Geometry check sheet. Reference: the model listing, model coordinates, mm. Face numbers are marked on the shaded views. A direction names the side the tool comes from. Give positions to 0.01 mm unless a question says otherwise; leave off trailing zeros. Write each loop counter-clockwise with the first axis right and the second up, starting at its lowest first coordinate (ties: lowest second). Pieces come first, ordered by that corner, then holes. Notation, with made-up numbers: M -37.5,18 L -32.5,18 A30 ccw -32.5,52 Z; hole C 19.25,74 d4. An arc over 180 degrees is marked long. Use one line per item in the form item = value. Start each with the question number.
```python
from build123d import *

# Parameters (mm, degrees)
F1_DEPTH  = 11.5
F3_R      = 2.75
F3_R_2    = 2.1
F4_DEPTH  = 7.2
F4_TAPER  = 1
F5_W      = 8.4
F5_H      = 28
F6_DEPTH  = 8
F8_DEPTH  = 15
F10_W     = 4.6
F10_H     = 5.4
F11_DEPTH = 20
F12_W     = 10.3
F12_H     = 7.2
F13_DEPTH = 10
F14_R     = 2
F15_DEPTH = 2
F16_R     = 2.1
F17_DEPTH = 2
F18_R     = 2.1
F19_DEPTH = 2
F20_R     = 2.1
F21_DEPTH = 2
F22_R     = 2.1
F23_DEPTH = 2
F24_R     = 2.1
F25_DEPTH = 2
F26_W     = 10.3
F26_H     = 7.2
F27_DEPTH = 10
F9_R      = 1.75
F28_DEPTH = 12
F29_R     = 1.5
F30_DEPTH = 0.8
F31_W     = 4.9
F31_H     = 8
F32_DEPTH = 1
F33_W     = 3
F33_H     = 1
F34_DEPTH = 5
F35_W     = 3
F35_H     = 1
F36_DEPTH = 5


with BuildPart() as f1:
    # F0 (on Front) → F1 (new body)
    with BuildSketch(Plane.XZ):
        Polygon((0.1941817731, -9.3541857075), (0.1941817731, 10.6458142925), (-6.1058182269, 10.6458142925), (-6.1058182269, 3.3958142925), (-9.7058182269, 3.3958142925), (-9.7058182269, 10.6458142925), (-16.0058182269, 10.6458142925), (-16.0058182269, 14.6458142925), (-29.7058182269, 14.6458142925), (-29.7058182269, 4.2458142925), (-31.1058182269, 4.2458142925), (-31.1058182269, -2.9541857075), (-29.7058182269, -2.9541857075), (-29.7058182269, -13.3541857075), (-16.0058182269, -13.3541857075), (-16.0058182269, -9.3541857075), (-9.7058182269, -9.3541857075), (-9.7058182269, -2.1041857075), (-6.1058182269, -2.1041857075), (-6.1058182269, -9.3541857075), align=None)
    extrude(amount=F1_DEPTH)

    # F3 (on face) → F4 (join)
    with BuildSketch(Plane.XZ.offset(11.5)):
        with Locations((-2.9558182269, 5.6458142925)):
            Circle(F3_R)
        with Locations((-2.9558182269, 5.6458142925)):
            Circle(F3_R_2, mode=Mode.SUBTRACT)
        with Locations((-2.9558182269, -4.3541857075)):
            Circle(F3_R)
        with Locations((-2.9558182269, -4.3541857075)):
            Circle(F3_R_2, mode=Mode.SUBTRACT)
        with Locations((-12.9558182269, 5.6458142925)):
            Circle(F3_R)
        with Locations((-12.9558182269, 5.6458142925)):
            Circle(F3_R_2, mode=Mode.SUBTRACT)
        with Locations((-12.9558182269, -4.3541857075)):
            Circle(F3_R)
        with Locations((-12.9558182269, -4.3541857075)):
            Circle(F3_R_2, mode=Mode.SUBTRACT)
        with Locations((-19.4558182269, -7.3541857075)):
            Circle(F3_R)
        with Locations((-19.4558182269, -7.3541857075)):
            Circle(F3_R_2, mode=Mode.SUBTRACT)
        with Locations((-19.4558182269, 8.6458142925)):
            Circle(F3_R)
        with Locations((-19.4558182269, 8.6458142925)):
            Circle(F3_R_2, mode=Mode.SUBTRACT)
    extrude(amount=F4_DEPTH, taper=F4_TAPER)

    # F5 (on face) → F6 (join)
    with BuildSketch(Plane.XZ.offset(11.5)):
        with Locations((-25.5058182269, 0.6458142925)):
            Rectangle(F5_W, F5_H)
    extrude(amount=F6_DEPTH)

    # F7 (on face) → F8 (cut)
    with BuildSketch(Plane.XZ.offset(19.5)):
        Polygon((-22.3058182269, 13.6458142925), (-28.7058182269, 13.6458142925), (-28.7058182269, 2.6458142925), (-29.2058182269, 2.6458142925), (-29.2058182269, -1.3541857075), (-28.7058182269, -1.3541857075), (-28.7058182269, -12.3541857075), (-22.3058182269, -12.3541857075), align=None)
    extrude(amount=-F8_DEPTH, mode=Mode.SUBTRACT)

    # F10 (on face) → F11 (cut, through all)
    with BuildSketch(Plane(origin=(0, 0, -9.3541857075), x_dir=(1, 0, 0), z_dir=(0, 0, -1))):
        with Locations((-3.1058182269, 7)):
            Rectangle(F10_W, F10_H)
        with Locations((-12.8558182269, 7)):
            Rectangle(F10_W, F10_H)
    extrude(amount=-F11_DEPTH, mode=Mode.SUBTRACT)

    # F12 (on face) → F13 (cut)
    with BuildSketch(Plane(origin=(0, 0, -13.3541857075), x_dir=(1, 0, 0), z_dir=(0, 0, -1))):
        with Locations((-22.0558182269, 7.1)):
            Rectangle(F12_W, F12_H)
    extrude(amount=-F13_DEPTH, mode=Mode.SUBTRACT)

    # F14 (on face) → F15 (cut)
    with BuildSketch(Plane.XZ.offset(11.5)):
        with Locations((-12.9558182269, 5.6458142925)):
            Circle(F14_R)
    extrude(amount=-F15_DEPTH, mode=Mode.SUBTRACT)

    # F16 (on face) → F17 (cut)
    with BuildSketch(Plane.XZ.offset(11.5)):
        with Locations((-12.9558182269, -4.3541857075)):
            Circle(F16_R)
    extrude(amount=-F17_DEPTH, mode=Mode.SUBTRACT)

    # F18 (on face) → F19 (cut)
    with BuildSketch(Plane.XZ.offset(11.5)):
        with Locations((-2.9558182269, 5.6458142925)):
            Circle(F18_R)
    extrude(amount=-F19_DEPTH, mode=Mode.SUBTRACT)

    # F20 (on face) → F21 (cut)
    with BuildSketch(Plane.XZ.offset(11.5)):
        with Locations((-2.9558182269, -4.3541857075)):
            Circle(F20_R)
    extrude(amount=-F21_DEPTH, mode=Mode.SUBTRACT)

    # F22 (on face) → F23 (cut)
    with BuildSketch(Plane.XZ.offset(11.5)):
        with Locations((-19.4558182269, 8.6458142925)):
            Circle(F22_R)
    extrude(amount=-F23_DEPTH, mode=Mode.SUBTRACT)

    # F24 (on face) → F25 (cut)
    with BuildSketch(Plane.XZ.offset(11.5)):
        with Locations((-19.4558182269, -7.3541857075)):
            Circle(F24_R)
    extrude(amount=-F25_DEPTH, mode=Mode.SUBTRACT)

    # F26 (on face) → F27 (cut)
    with BuildSketch(Plane.XY.offset(14.6458142925)):
        with Locations((-22.0558182269, -7.1)):
            Rectangle(F26_W, F26_H)
    extrude(amount=-F27_DEPTH, mode=Mode.SUBTRACT)

    # F9 (on face) → F28 (cut)
    with BuildSketch(Plane.XZ.offset(11.5)):
        with Locations((-7.9058182269, 0.6458142925)):
            Circle(F9_R)
        with Locations((-12.9058182269, 0.6458142925)):
            Circle(F9_R)
        with Locations((-17.9058182269, 0.6458142925)):
            Circle(F9_R)
    extrude(amount=-F28_DEPTH, mode=Mode.SUBTRACT)

    # F29 (on face) → F30 (join)
    with BuildSketch(Plane(origin=(0, 0, 0), x_dir=(-1, 0, 0), z_dir=(0, 1, 0))):
        with Locations((27.9058182269, 0.6458142925)):
            Circle(F29_R)
    extrude(amount=F30_DEPTH)

    # F31 (on face) → F32 (cut, through all)
    with BuildSketch(Plane.XZ.offset(4.5)):
        with Locations((-24.7558182269, 0.6458142925)):
            Rectangle(F31_W, F31_H)
    extrude(amount=-F32_DEPTH, mode=Mode.SUBTRACT)

    # F33 (on face) → F34 (join)
    with BuildSketch(Plane(origin=(0, -10.7, 0), x_dir=(-1, 0, 0), z_dir=(0, 1, 0))):
        with Locations((23.9058182269, -12.8541857075)):
            Rectangle(F33_W, F33_H)
    extrude(amount=F34_DEPTH)

    # F35 (on face) → F36 (join)
    with BuildSketch(Plane(origin=(0, -10.7, 0), x_dir=(-1, 0, 0), z_dir=(0, 1, 0))):
        with Locations((23.9058182269, 14.1458142925)):
            Rectangle(F35_W, F35_H)
    extrude(amount=F36_DEPTH)


solid = f1.part
```
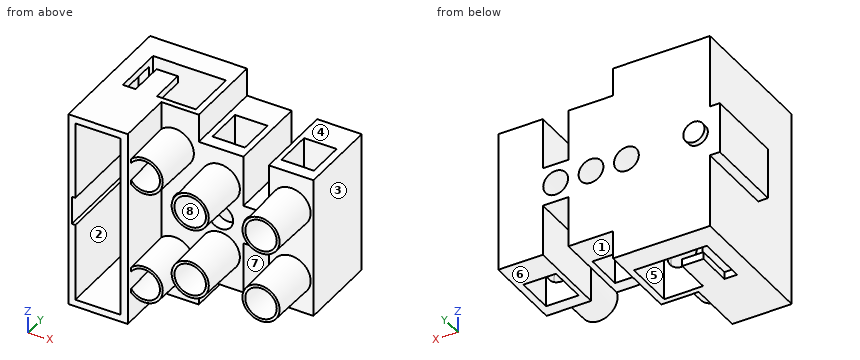
(1) Sectioned sample at B-B, the plane y = -13.75. State how many separate pieces and enclosed holes the cut face has, plus the area to 3 significant figures.
(2) Draft check along X on the marked faces 1, 2 and 3. Enter one of: released by +X, released by -X, zero draft, split by the parting line, or undercut.
(3) Tool access check on the marked faces 4, 5, 6, 7 and 8. Record the directions out of +Z, -Z, +X, -X, +Y, -Y that give a thin tool (end or side, any length) a straight path to the whole face; none if there is none.
(4) Sectioned sample at A-A, the plane x = -26. Record the boundary of the cut face in (y, z).
(5) Depth check by flat-ended pin: pin 1 (8 mm diameter, centred on x = -18, z = 5.5, fed in from +Y); pin 2 (5 mm diameter, centred on x = -18.5, z = -6.5, fed in from -Y); pin 3 (3.5 mm diameter, centred on x = -19.46, z = 8.65, fed in from -Y). Enter the tip coordinate at first touch or a pass-through.
(6) Sectioned sample at C-C, the plane y = -3. Record the boundary of the cut face in (x, z), plus the area to 3 significant figures.
(7) Thickness scan on probe 1 along X at (y, z) = (-4, 6.25); probe 2 along Z at (x, y) = (-13.5, -15.75); probe 3 along X at (y, z) = (-8.5, -2.75). Record the ranges inside material, lowest first. Write a range as [from, to].
Numbers:
q1.separate_pieces = 5
q1.enclosed_holes = 7
q1.area = 115 mm2
q2.face_1 = zero draft
q2.face_2 = undercut
q2.face_3 = released by +X
q3.face_4 = +Z, +X, +Y, -Y
q3.face_5 = -Z
q3.face_6 = -Z, +X, +Y, -Y
q3.face_7 = -Z, +Y, -Y
q3.face_8 = -Y
q4.outline = M -19.5,-13.35 L -10.7,-13.35 L -10.7,-12.35 L -19.5,-12.35 Z; M -19.5,13.65 L -10.7,13.65 L -10.7,14.65 L -19.5,14.65 Z; M -3.5,-13.35 L 0,-13.35 L 0,14.65 L -3.5,14.65 Z
q5.pin_1 = 0
q5.pin_2 = -18.7
q5.pin_3 = -3.5
q6.outline = M -31.11,-2.95 L -29.71,-2.95 L -29.71,-13.35 L -16.01,-13.35 L -16.01,-9.35 L -9.71,-9.35 L -9.71,-2.1 L -6.11,-2.1 L -6.11,-9.35 L 0.19,-9.35 L 0.19,10.65 L -6.11,10.65 L -6.11,3.4 L -9.71,3.4 L -9.71,10.65 L -16.01,10.65 L -16.01,14.65 L -29.71,14.65 L -29.71,4.25 L -31.11,4.25 Z; hole C -17.91,0.65 d3.5; hole C -12.91,0.65 d3.5; hole C -7.91,0.65 d3.5
q6.area = 637 mm2
q7.probe_1 = [-29.71, -27.21], [-16.91, -9.71], [-6.11, 0.19]
q7.probe_2 = [-6.97, -6.46], [-2.25, -1.73], [3.03, 3.54], [7.75, 8.27]
q7.probe_3 = [-31.11, -28.71], [-22.31, -15.16], [-10.56, -9.71], [-6.11, -5.41], [-0.81, 0.19]
